```python
from build123d import *

# Parameters (mm, degrees)
BOSS_EXTRUDE1_DEPTH = 162.5
SKETCH2_R           = 1.25
CUT_EXTRUDE1_DEPTH  = 8
CUT_EXTRUDE2_DEPTH  = 1
SKETCH4_R           = 1.25
CUT_EXTRUDE3_DEPTH  = 3


with BuildPart() as part:
    # Sketch1 → Boss-Extrude1 (new body)
    with BuildSketch(Plane.XY):
        Polygon((0, 9), (0, -9), (7, -9), (7, -7), (2, -7), (2, 7), (7, 7), (7, 9), align=None)
    extrude(amount=-BOSS_EXTRUDE1_DEPTH)

    # Sketch2 → Cut-Extrude1 (cut, through all)
    with BuildSketch(Plane.ZY):
        with Locations((-5, 3)):
            Circle(SKETCH2_R)
        with Locations((-5, -3)):
            Circle(SKETCH2_R)
        with Locations((-157.5, -3)):
            Circle(SKETCH2_R)
        with Locations((-157.5, 3)):
            Circle(SKETCH2_R)
    extrude(amount=-CUT_EXTRUDE1_DEPTH, mode=Mode.SUBTRACT)

    # Sketch3 → Cut-Extrude2 (cut)
    with BuildSketch(Plane.ZY):
        Polygon((-8.84619024, 4.575146227), (-7.141062035, 4.575146227), (-7.141062035, 4.216171868), (-8.532087676, 4.216171868), (-8.532087676, 3.139248791), (-7.141062035, 3.139248791), (-7.141062035, 2.780274432), (-8.532087676, 2.780274432), (-8.532087676, 1.075146227), (-8.84619024, 1.075146227), align=None)
    extrude(amount=-CUT_EXTRUDE2_DEPTH, mode=Mode.SUBTRACT)

    # Sketch4 → Cut-Extrude3 (cut)
    with BuildSketch(Plane.XZ.offset(9)):
        with Locations((4.5, -37)):
            Circle(SKETCH4_R)
        with Locations((4.5, -43)):
            Circle(SKETCH4_R)
        with Locations((4.5, -112)):
            Circle(SKETCH4_R)
        with Locations((4.5, -118)):
            Circle(SKETCH4_R)
    extrude(amount=-CUT_EXTRUDE3_DEPTH, mode=Mode.SUBTRACT)


solid = part.part
```
Verification items for the finished model (mm, model axes). A direction names the side the tool comes from. Coordinates: 2 decimals unless noted, no trailing zeros. Loops run counter-clockwise (first coordinate to the right, second up) from the corner with the lowest first, then second, coordinate; pieces in that order, holes last. Notation, with made-up numbers: (24.5, 57) - (63.5, 57) arc R29 ccw to (63.5, 88) - close; hole circle Ø10 at (88, 32.5). An arc over 180 degrees is marked (long way). Answer as a JSON object with one key per item and string values.
(1) Cross-section at B-B, the plane z = -48. Record the boundary of the cut face in (x, y).
Response:
{"outline": "(0, -9) - (7, -9) - (7, -7) - (2, -7) - (2, 7) - (7, 7) - (7, 9) - (0, 9) - close"}
(2) Cross-section at A-A, the plane x = 4.5. Record the boundary of the cut face in (y, z), then the cut area to 3 significant figures.
Response:
{"outline": "(-9, -162.5) - (-7, -162.5) - (-7, -119.25) - (-9, -119.25) - close; (-9, -116.75) - (-7, -116.75) - (-7, -113.25) - (-9, -113.25) - close; (-9, -110.75) - (-7, -110.75) - (-7, -44.25) - (-9, -44.25) - close; (-9, -41.75) - (-7, -41.75) - (-7, -38.25) - (-9, -38.25) - close; (-9, -35.75) - (-7, -35.75) - (-7, 0) - (-9, 0) - close; (7, -162.5) - (9, -162.5) - (9, 0) - (7, 0) - close", "area": "630 mm²"}
(3) Access from +Z, -Z, +X, -X, +Y, -Y to the whole of each face (thin tool, end or side, straight path). Record for faces 1 (the flat face through (4, 7, -80)), 2 (the cylindrical face through (4.34, -8.01, -116.76)), 3 (the cylindrical face through (0.986, -3.479, -156.345)).
Response:
{"face 1": "+Z, -Z, +X", "face 2": "-Y", "face 3": "+X, -X"}
(4) Go/stop test with flat-tipped pins: pin 1 Ø3 at (y, z) = (1.5, -83) entering from +X; pin 2 Ø2 at (x, z) = (4.5, -118) entering from -Y. Record where each tip stops, or that it passes through.
Response:
{"pin 1": "stops at x = 2", "pin 2": "stops at y = 7"}
(5) Scan lines: line 1 along Y through (x, z) = (0.5, -157.5); line 2 along Z through (x, y) = (4.5, -8.5); line 3 along Z through (x, y) = (1.75, 2.75). Record each from-to range of solid material in increasing order.
Response:
{"line 1": "y = -9 to -4.25, -1.75 to 1.75, 4.25 to 9", "line 2": "z = -162.5 to -119.25, -116.75 to -113.25, -110.75 to -44.25, -41.75 to -38.25, -35.75 to 0", "line 3": "z = -162.5 to -158.72, -156.28 to -6.22, -3.78 to 0"}
(6) Mould release check, pull along Y, two halves, no side actions. Record for faces 4 (the cylindrical face through (4.23, -8.01, -38.22)), 5 (the cylindrical face through (0.986, 2.521, -156.345)), 6 (the flat face through (3, -9, -80)): pulls with the +Y half, pulls with the -Y half, needs draft (parallel to the pull), parting line crosses it, or undercut.
Response:
{"face 4": "needs draft", "face 5": "undercut", "face 6": "pulls with the -Y half"}
